Could you check a few things on this model? Use its own coordinates, in mm. Face numbers are marked on the shaded views. A direction names the side the tool comes from. Round coordinates to 2 decimals unless told otherwise and drop trailing zeros. Loops run counter-clockwise (first coordinate to the right, second up) from the corner with the lowest first, then second, coordinate; pieces in that order, holes last. Notation, with made-up numbers: (-16.75, -2) -> (-12.75, -2) arc R22 ccw to (-12.75, 13) -> close; hole circle Ø8 at (-34, 86). An arc over 180 degrees is marked (long way). One line per item, written item: value.
from build123d import *

# Parameters (mm, degrees)
SKETCH2_W           = 76
SKETCH2_H           = 20
SKETCH2_R           = 0.75
BOSS_EXTRUDE1_DEPTH = 2
SKETCH3_W           = 76
SKETCH3_H           = 15
SKETCH3_R           = 0.75
BOSS_EXTRUDE2_DEPTH = 2


with BuildPart() as part:
    # Sketch2 → Boss-Extrude1 (new body)
    with BuildSketch(Plane.XY):
        with Locations((38, 10)):
            Rectangle(SKETCH2_W, SKETCH2_H)
        with Locations((44, 17.5)):
            Circle(SKETCH2_R, mode=Mode.SUBTRACT)
        with Locations((56, 17.5)):
            Circle(SKETCH2_R, mode=Mode.SUBTRACT)
        with Locations((68, 17.5)):
            Circle(SKETCH2_R, mode=Mode.SUBTRACT)
        with Locations((32, 17.5)):
            Circle(SKETCH2_R, mode=Mode.SUBTRACT)
        with Locations((20, 17.5)):
            Circle(SKETCH2_R, mode=Mode.SUBTRACT)
        with Locations((8, 17.5)):
            Circle(SKETCH2_R, mode=Mode.SUBTRACT)
    extrude(amount=BOSS_EXTRUDE1_DEPTH)

    # Sketch3 → Boss-Extrude2 (add)
    with BuildSketch(Plane(origin=(0, 0, 0), x_dir=(-1, 0, 0), z_dir=(0, -1, 0))):
        with Locations((-38, -7.5)):
            Rectangle(SKETCH3_W, SKETCH3_H)
        with Locations((-13, -10)):
            Circle(SKETCH3_R, mode=Mode.SUBTRACT)
        with Locations((-23, -10)):
            Circle(SKETCH3_R, mode=Mode.SUBTRACT)
        with Locations((-33, -10)):
            Circle(SKETCH3_R, mode=Mode.SUBTRACT)
        with Locations((-43, -10)):
            Circle(SKETCH3_R, mode=Mode.SUBTRACT)
        with Locations((-53, -10)):
            Circle(SKETCH3_R, mode=Mode.SUBTRACT)
        with Locations((-63, -10)):
            Circle(SKETCH3_R, mode=Mode.SUBTRACT)
    extrude(amount=BOSS_EXTRUDE2_DEPTH)


solid = part.part
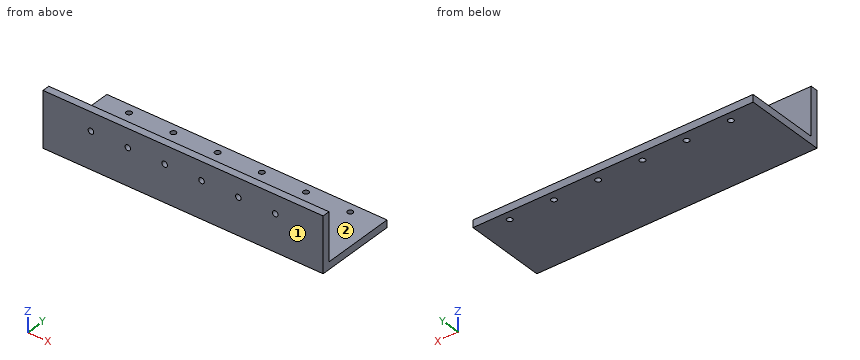
(1) If we section it at B-B, the plane y = 11: Please give me the cut outline in (x, z).
Recorded:
outline: (0, 0) -> (76, 0) -> (76, 2) -> (0, 2) -> close
(2) If we section it at D-D, the plane z = 13.5: Please give me the cut outline in (x, y), then the cut area to 3 significant figures.
Recorded:
outline: (0, -2) -> (76, -2) -> (76, 0) -> (0, 0) -> close
area: 152 mm²
(3) If we section it at A-A, the plane x = 63: Please give me the cut outline in (y, z).
Recorded:
outline: (-2, 0) -> (20, 0) -> (20, 2) -> (0, 2) -> (0, 9.25) -> (-2, 9.25) -> close; (-2, 10.75) -> (0, 10.75) -> (0, 15) -> (-2, 15) -> close
(4) I'm going to push flat-ended pins straight in: pin 1 Ø6.5 at (x, z) = (26.5, 11.5) entering from +Y; pin 2 Ø1.7 at (x, y) = (8, 17.5) entering from +Z; pin 3 Ø8 at (x, z) = (16, 5) entering from +Y; pin 4 Ø1.4 at (x, z) = (23, 10) entering from +Y. Where does each tip first touch, or does it pass through?
Recorded:
pin 1: y = 0
pin 2: z = 2
pin 3: y = 20
pin 4: through
(5) For the marked faces 1 and 2, which set-ups out of +Z, -Z, +X, -X, +Y, -Y let a thin tool reach every point of the face, with its end or its side?
Recorded:
face 1: +Z, -Z, +X, -X, -Y
face 2: +Z, +X, -X, +Y
(6) If I drill on L1, parallel to Y at x = 68, z = 0.95; L2, parallel to Z at x = 53, y = -1.05; L3, parallel to Z at x = 68, y = 9.25, over which ranges is the centre line in solid material (lowest first)?
Recorded:
L1: -2 to 16.75, 18.25 to 20
L2: 0 to 9.25, 10.75 to 15
L3: 0 to 2
(7) If we section it at C-C, the plane x = 49: Please give me the cut outline in (y, z), then the cut area to 3 significant figures.
Recorded:
outline: (-2, 0) -> (20, 0) -> (20, 2) -> (0, 2) -> (0, 15) -> (-2, 15) -> close
area: 70.0 mm²
